Work out the finished part from the listing and answer in its coordinate system (mm). Face numbers are marked on the shaded views. A direction names the side the tool comes from. Coordinates: 2 decimals unless noted, no trailing zeros. Write each loop counter-clockwise with the first axis right and the second up, starting at its lowest first coordinate (ties: lowest second). Pieces come first, ordered by that corner, then holes. Notation, with made-up numbers: (7.5, 14.5) - (62.5, 14.5) arc R17 ccw to (62.5, 41.5) - close; hole circle Ø6 at (-12, 3.25). An arc over 180 degrees is marked (long way). Answer as a JSON object with one key per item and string values. Group by question number.
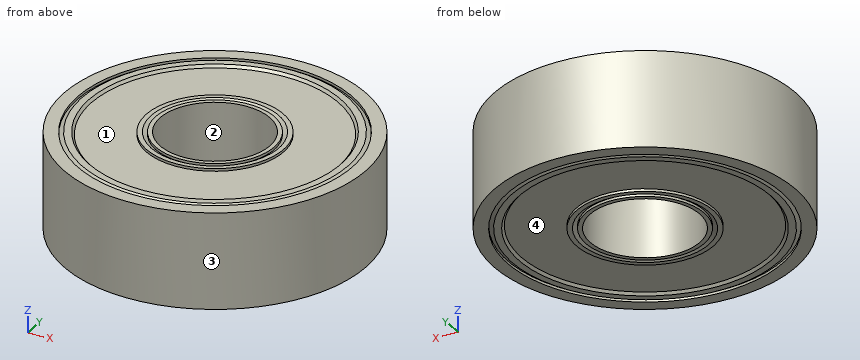
from build123d import *

# Parameters (mm, degrees)
SKETCH1_R           = 11
SKETCH1_R_2         = 4
BOSS_EXTRUDE1_DEPTH = 7


with BuildPart() as part:
    # Sketch1 → Boss-Extrude1 (new body)
    with BuildSketch(Plane.XY):
        Circle(SKETCH1_R)
        Circle(SKETCH1_R_2, mode=Mode.SUBTRACT)
    extrude(amount=BOSS_EXTRUDE1_DEPTH)

    # Sketch2 → Cut-Revolve1 (revolve, cut)
    with BuildSketch(Plane(origin=(0, 0, 0), x_dir=(1, 0, 0), z_dir=(0, 1, 0))):
        Polygon((-9, -6.809352766), (-5, -6.809352766), (-5, -7.059352766), (-4.645185355, -7), (-4.319740766, -6.809352766), (-4.319740766, -7), (0, -7), (0, -9.290623362), (-10.991354846, -9.290623362), (-10.991354846, -7.309352766), (-10.001460887, -7.309352766), (-10.001460887, -6.809352766), (-9.350571708, -7.202353914), align=None)
        Polygon((-4.645185355, 0), (-5, 0.059352766), (-5, -0.190647234), (-9, -0.190647234), (-9.350571708, 0.202353914), (-10.001460887, -0.190647234), (-10.001460887, 0.309352766), (-10.991354846, 0.309352766), (-10.991354846, 2.290623362), (0, 2.290623362), (0, 0), (-4.319740766, 0), (-4.319740766, -0.190647234), align=None)
    revolve(axis=Axis((0, 0, 0), (0, 0, 1)), mode=Mode.SUBTRACT)


solid = part.part
Q1. For a pull along X with two mould halves and no side action, classify the marked faces 3 and 4 as +X half, -X half, draft (parallel to the pull), parting line (faces both ways), or undercut.
Q2. Flat-ended cylindrical pins translate along their axes: pin 1 Ø9 at (x, y) = (0, 0) entering from +Z; pin 2 Ø3 at (y, z) = (-5.5, 6) entering from +X; pin 3 Ø1.5 at (x, y) = (-4, 4.5) entering from -Z; pin 4 Ø1.5 at (y, z) = (1, 4) entering from +X. Find the tip coordinate at first contact, or state that the pin passes through.
Q3. Section A-A on z = 5.5 is taken. Determine the outline of the cut face in (x, y), plus the area to 3 significant figures.
Q4. Consider L1, parallel to Y at x = 0, z = 5.75; L2, parallel to Z at x = -4, y = 6; L3, parallel to Y at x = 2.25, z = 3.5. Determine where each line is inside the solid, lowest interval first. Write a range as from..to.
Q5. A tool of negligible diameter and unlimited length cuts with its end or side. For the marked faces 1 and 2, from which of +Z, -Z, +X, -X, +Y, -Y can it reach the whole face along a straight path? Write none if from no direction.
Numbers:
{
 "1": {"face 3": "parting line", "face 4": "undercut"},
 "2": {"pin 1": "stops at z = 7", "pin 2": "stops at x = 10.25", "pin 3": "stops at z = 0.19", "pin 4": "stops at x = 11"},
 "3": {"outline": "circle Ø22 at (0, 0); hole circle Ø8 at (0, 0)", "area": "330 mm²"},
 "4": {"L1": "y = -11..-4, 4..11", "L2": "z = 0.19..6.81", "L3": "y = -10.77..-3.31, 3.31..10.77"},
 "5": {"face 1": "+Z", "face 2": "+Z, -Z"}
}
